```python
from build123d import *

# Parameters (mm, degrees)
SKETCH1_R           = 40
BOSS_EXTRUDE1_DEPTH = 5
SKETCH2_R           = 32.5
BOSS_EXTRUDE2_DEPTH = 5
SKETCH6_W           = 20
SKETCH6_H           = 20
BOSS_EXTRUDE3_DEPTH = 20
CUT_EXTRUDE15_DEPTH = 85.403791384
CUT_EXTRUDE16_DEPTH = 85.40379142
CUT_EXTRUDE22_DEPTH = 85.40379142
CUT_EXTRUDE23_DEPTH = 85.40379142


with BuildPart() as part:
    # Sketch1 → Boss-Extrude1 (new body)
    with BuildSketch(Plane(origin=(0, 0, 0), x_dir=(1, 0, 0), z_dir=(0, 1, 0))):
        with Locations(Location((0, 0, 0), (0, 0, 270))):
            Circle(SKETCH1_R)
    extrude(amount=BOSS_EXTRUDE1_DEPTH)

    # Sketch2 → Boss-Extrude2 (add)
    with BuildSketch(Plane(origin=(0, 5, 0), x_dir=(1, 0, 0), z_dir=(0, 1, 0))):
        with Locations(Location((0, 0, 0), (0, 0, 270))):
            Circle(SKETCH2_R)
    extrude(amount=BOSS_EXTRUDE2_DEPTH)

    # Sketch6 → Boss-Extrude3 (add)
    with BuildSketch(Plane(origin=(0, 10, 0), x_dir=(1, 0, 0), z_dir=(0, 1, 0))):
        Polygon((-5, -28), (5, -28), (10, -10), (-10, -10), align=None)
        Polygon((28, -5), (28, 5), (10, 10), (10, -10), align=None)
        Polygon((5, 28), (-5, 28), (-10, 10), (10, 10), align=None)
        Polygon((-28, 5), (-28, -5), (-10, -10), (-10, 10), align=None)
        Rectangle(SKETCH6_W, SKETCH6_H)
    extrude(amount=BOSS_EXTRUDE3_DEPTH)

    # Sketch12 → Cut-Extrude15 (cut, through all)
    with BuildSketch(Plane(origin=(0, 0, -28), x_dir=(-1, 0, 0), z_dir=(0, 0, -1))):
        with BuildLine():
            Line((-28, 30), (-28, 12))
            add(Edge.make_bspline(
                [(-12, 30), (-16.636316338, 12.206521784), (-28, 12)],
                knots=[0, 0, 0, 0.849765105, 0.849765105, 0.849765105], degree=2))
            Line((-12, 30), (-28, 30))
        make_face()
        with BuildLine():
            add(Edge.make_bspline(
                [(12, 30), (16.636316338, 12.206521784), (28, 12)],
                knots=[0, 0, 0, 0.849765105, 0.849765105, 0.849765105], degree=2))
            Line((28, 12), (28, 30))
            Line((28, 30), (12, 30))
        make_face()
    extrude(amount=-CUT_EXTRUDE15_DEPTH, mode=Mode.SUBTRACT)

    # Sketch13 → Cut-Extrude16 (cut, through all)
    with BuildSketch(Plane(origin=(28, 0, 0), x_dir=(0, 0, -1), z_dir=(1, 0, 0))):
        with BuildLine():
            Line((-28, 30), (-28, 12))
            add(Edge.make_bspline(
                [(-12, 30), (-16.636316338, 12.206521784), (-28, 12)],
                knots=[0, 0, 0, 0.849765105, 0.849765105, 0.849765105], degree=2))
            Line((-12, 30), (-28, 30))
        make_face()
        with BuildLine():
            add(Edge.make_bspline(
                [(12, 30), (16.636316338, 12.206521784), (28, 12)],
                knots=[0, 0, 0, 0.849765105, 0.849765105, 0.849765105], degree=2))
            Line((28, 12), (28, 30))
            Line((28, 30), (12, 30))
        make_face()
    extrude(amount=-CUT_EXTRUDE16_DEPTH, mode=Mode.SUBTRACT)

    # Sketch15 → Cut-Extrude22 (cut, through all)
    with BuildSketch(Plane.XY.offset(28)):
        with BuildLine():
            ThreePointArc((-3.5, 30), (0, 26.5), (3.5, 30))
            Line((3.5, 30), (-3.5, 30))
        make_face()
    extrude(amount=-CUT_EXTRUDE22_DEPTH, mode=Mode.SUBTRACT)

    # Sketch16 → Cut-Extrude23 (cut, through all)
    with BuildSketch(Plane(origin=(28, 0, 0), x_dir=(0, 0, -1), z_dir=(1, 0, 0))):
        with BuildLine():
            ThreePointArc((-8, 30), (0, 22), (8, 30))
            Line((8, 30), (-8, 30))
        make_face()
    extrude(amount=-CUT_EXTRUDE23_DEPTH, mode=Mode.SUBTRACT)


solid = part.part
```
Source: CAD feature listing. Evaluate the final solid. Frame: model axes, mm. A direction names the side the tool comes from. Round coordinates to 2 decimals unless told otherwise and drop trailing zeros. Loops run counter-clockwise (first coordinate to the right, second up) from the corner with the lowest first, then second, coordinate; pieces in that order, holes last.
(1) Section query B-B (z = -30). Output: boundary loops of the cut face in (x, y), and give its area (3 significant figures).
From the geometry:
outline: (-26.46, 0) - (26.46, 0) - (26.46, 5) - (12.5, 5) - (12.5, 10) - (-12.5, 10) - (-12.5, 5) - (-26.46, 5) - close
area: 390 mm2
(2) Access query for faces 1 (the flat face through (33, 5, 0)), 2 (the flat face through (14.874, 15.416, 8.646)), 3 (the flat face through (-28, 11, 0)). Directions: +Z, -Z, +X, -X, +Y, -Y. A direction counts if a zero-diameter tool reaches every point of the face in a straight line with its end or side. Return the directions, or none.
From the geometry:
face 1: +Y
face 2: +Z, +X, +Y
face 3: +Z, -Z, -X, +Y
(3) Section query A-A (y = 4). Output: boundary loops of the cut face in (x, z), and give its area (3 significant figures).
From the geometry:
outline: circle Ø80 at (0, 0)
area: 5,030 mm2
(4) Pull-direction query (Z, two-part tool) for faces 4 (the cylindrical face through (-0.1, 26.5, -10.1)), 5 (the flat face through (-8.646, 15.416, 14.874)), 6 (the flat face through (0, 11, -28)), 7 (the cylindrical face through (0, 22, 0)); classes: +Z half, -Z half, draft (parallel to the pull), parting line (faces both ways), or undercut.
From the geometry:
face 4: draft
face 5: +Z half
face 6: -Z half
face 7: undercut
(5) Material intervals for probe 1 along Y at (x, z) = (-30.5, -18.5); probe 2 along Y at (x, z) = (-13, -15); probe 3 along Z at (x, y) = (12, 21.5), sorted ascending.
From the geometry:
probe 1: y = 0 to 5
probe 2: y = 0 to 10
probe 3: z = -9.44 to 9.44
(6) Contact query for flat-ended pins moving along their axis: pin 1 Ø0.6 at (y, z) = (10.5, 0) entering from -X; pin 2 Ø1.5 at (y, z) = (3.5, 22.5) entering from +X; pin 3 Ø1 at (x, y) = (5, 7.5) entering from -Z. Output: stop coordinate, or through.
From the geometry:
pin 1: stops at x = -28
pin 2: stops at x = 33.57
pin 3: stops at z = -32.19
